For this review, take the finished solid that the model builds, in its own axes (mm). A direction names the side the tool comes from. Round coordinates to 2 decimals unless told otherwise and drop trailing zeros. Loops run counter-clockwise (first coordinate to the right, second up) from the corner with the lowest first, then second, coordinate; pieces in that order, holes last. Notation, with made-up numbers: (55, 55.25) -> (75, 55.25) arc R30 ccw to (75, 83.25) -> close; hole circle Ø3 at (69, -9.5). An arc over 180 degrees is marked (long way). One line per question, with ' | ' between items. Start each with the question number.
1. Draft analysis for pull direction X (two halves, no side actions). For faces 4 (the face through (-110.065, 60.626, 3.131)), 5 (the face through (-2, 188, 6.35)), 6 (the face through (92.08, 139.35, 3.13)), state which applies: pulls with the +X half, pulls with the -X half, needs draft (parallel to the pull), parting line crosses it, or undercut.
2. Consider section A-A (y = 144.5). Write out the cut boundary in (x, z).
3. Wall thickness on line 1 along X through (y, z) = (227.5, 3.25); line 2 along X through (y, z) = (77, 4.5); line 3 along X through (y, z) = (84.5, 2): over which ranges is each line inside the solid? List them lowest first.
4. Consider section B-B (x = -79.5). Write out the cut boundary in (y, z), and give its area (3 significant figures).
5. For faces 1 (the face through (61.4, 281.5, 3.1)), 2 (the face through (49.2, 90.5, 3.1)), 3 (the face through (-88.054, 83.517, 3.131)), list the 3-axis set-ups (+Z, -Z, +X, -X, +Y, -Y) from which the entire face can be reached by the end or side of a thin tool; tool diameter is ignored.
6. For pin 1 Ø3 at (x, z) = (126.5, 4.5) entering from -Y; pin 2 Ø1 at (y, z) = (219, 3.5) entering from +X; pin 3 Ø3 at (y, z) = (273.5, 2.5) entering from +X; pin 4 Ø3 at (x, y) = (-120.5, 99.5) entering from +Z, all flat-tipped, find the tip position at first contact; note any pin that passes through.
```python
from build123d import *

# Parameters (mm, degrees)
F1_DEPTH = 6.35


with BuildPart() as f1:
    # F0 (on Top) → F1 (new body)
    with BuildSketch(Plane.XY):
        with BuildLine():
            Line((-152.4, 123.825), (-152.4, 0))
            Line((-152.4, 0), (-139.7, 0))
            Line((-139.7, 0), (-94.56907, 45.13093))
            Line((-94.56907, 45.13093), (-125.999967, 76.561826))
            ThreePointArc((-125.999967, 76.561826), (-125.999967, 99.012467), (-103.549326, 99.012467))
            Line((-103.549326, 99.012467), (-72.11843, 67.58157))
            Line((-72.11843, 67.58157), (-26.9875, 112.7125))
            Line((-26.9875, 112.7125), (-26.9875, 158.75))
            ThreePointArc((-26.9875, 158.75), (0, 185.7375), (26.9875, 158.75))
            Line((26.9875, 158.75), (26.9875, 112.7125))
            Line((26.9875, 112.7125), (72.11843, 67.58157))
            Line((72.11843, 67.58157), (103.549326, 99.012467))
            ThreePointArc((103.549326, 99.012467), (120.849746, 102.453734), (130.649646, 87.787146))
            ThreePointArc((130.649646, 87.787146), (129.441234, 81.712047), (125.999967, 76.561826))
            Line((125.999967, 76.561826), (94.56907, 45.13093))
            Line((94.56907, 45.13093), (139.7, 0))
            Line((139.7, 0), (152.4, 0))
            Line((152.4, 0), (152.4, 123.825))
            Line((152.4, 123.825), (107.95, 123.825))
            ThreePointArc((107.95, 123.825), (92.075, 139.7), (107.95, 155.575))
            Line((107.95, 155.575), (152.4, 155.575))
            Line((152.4, 155.575), (152.4, 190.5))
            Line((152.4, 190.5), (106.47532, 236.42468))
            Line((106.47532, 236.42468), (75.044424, 204.993783))
            ThreePointArc((75.044424, 204.993783), (52.593783, 204.993783), (52.593783, 227.444424))
            Line((52.593783, 227.444424), (84.02468, 258.87532))
            Line((84.02468, 258.87532), (38.1, 304.8))
            Line((38.1, 304.8), (15.875, 304.8))
            Line((15.875, 304.8), (15.875, 260.35))
            ThreePointArc((15.875, 260.35), (0, 244.475), (-15.875, 260.35))
            Line((-15.875, 260.35), (-15.875, 304.8))
            Line((-15.875, 304.8), (-38.1, 304.8))
            Line((-38.1, 304.8), (-84.02468, 258.87532))
            Line((-84.02468, 258.87532), (-52.593783, 227.444424))
            ThreePointArc((-52.593783, 227.444424), (-52.593783, 204.993783), (-75.044424, 204.993783))
            Line((-75.044424, 204.993783), (-106.47532, 236.42468))
            Line((-106.47532, 236.42468), (-152.4, 190.5))
            Line((-152.4, 190.5), (-152.4, 155.575))
            Line((-152.4, 155.575), (-107.95, 155.575))
            ThreePointArc((-107.95, 155.575), (-96.72468, 150.92532), (-92.075, 139.7))
            ThreePointArc((-92.075, 139.7), (-96.72468, 128.47468), (-107.95, 123.825))
            Line((-107.95, 123.825), (-152.4, 123.825))
        make_face()
    extrude(amount=F1_DEPTH)


solid = f1.part
```
Answer block:
1) face 4: undercut | face 5: needs draft | face 6: pulls with the +X half
2) outline: (-92.82, 0) -> (-26.99, 0) -> (-26.99, 6.35) -> (-92.82, 6.35) -> close; (26.99, 0) -> (92.82, 0) -> (92.82, 6.35) -> (26.99, 6.35) -> close
3) line 1: x = -115.4 to -97.55, -52.65 to 52.65, 97.55 to 115.4 | line 2: x = -152.4 to -126.42, -81.54 to -62.7, 62.7 to 81.54, 126.42 to 152.4 | line 3: x = -152.4 to -130.31, -89.04 to -55.2, 55.2 to 89.04, 130.31 to 152.4
4) outline: (74.96, 0) -> (209.45, 0) -> (209.45, 6.35) -> (74.96, 6.35) -> close; (254.35, 0) -> (263.4, 0) -> (263.4, 6.35) -> (254.35, 6.35) -> close | area: 911 mm2
5) face 1: +Z, -Z, +X, +Y | face 2: +Z, -Z, -Y | face 3: +Z, -Z
6) pin 1: stops at y = 11.7 | pin 2: stops at x = 124.4 | pin 3: stops at x = 70.9 | pin 4: passes through
